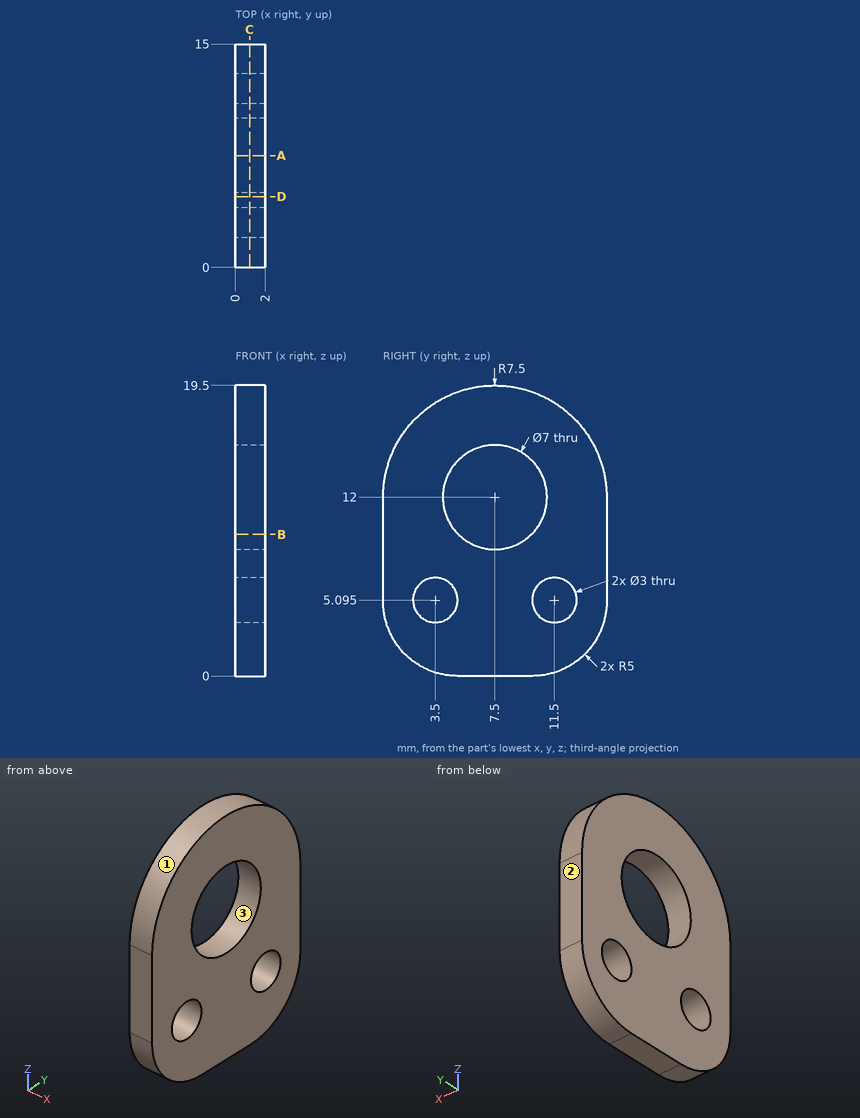
Study the drawing (mm; zero at the part's minimum x, y, z) and answer. Give positions to 0.01 mm unless a question says otherwise; leave off trailing zeros. Order: outer loops, then holes, each group sorted by start corner. A loop starts at its lowest first (then second) coordinate and runs counter-clockwise, first axis right, second up. Notation, with made-up numbers: (-2.5, 54.5) -> (37.5, 54.5) arc R29 cw to (37.5, 80.5) -> close; hole circle Ø8 at (43.5, 54.5). An arc over 180 degrees is marked (long way). Put each result on its own line as item: value.
Item 1: A cutting plane is placed at D-D on y = 4.75. Give the vertices of the cut face in (x, z) (1 decimal).
Established:
outline: (0, 0) -> (2, 0) -> (2, 4.3) -> (0, 4.3) -> close; (0, 5.9) -> (2, 5.9) -> (2, 9.8) -> (0, 9.8) -> close; (0, 14.2) -> (2, 14.2) -> (2, 19) -> (0, 19) -> close
Item 2: A cutting plane is placed at C-C on x = 0.95. Give the vertices of the cut face in (y, z) (3 decimals), plus the area to 3 significant figures.
Established:
outline: (0, 5) arc R5 ccw to (5, 0) -> (10, 0) arc R5 ccw to (15, 5) -> (15, 12) arc R7.5 ccw to (0, 12) -> close; hole circle Ø3 at (3.5, 5.095); hole circle Ø7 at (7.5, 12); hole circle Ø3 at (11.5, 5.095)
area: 205 mm^2
Item 3: A cutting plane is placed at A-A on y = 7.5. Give the vertices of the cut face in (x, z), plus the area to 3 significant figures.
Established:
outline: (0, 0) -> (2, 0) -> (2, 8.5) -> (0, 8.5) -> close; (0, 15.5) -> (2, 15.5) -> (2, 19.5) -> (0, 19.5) -> close
area: 25.0 mm^2
Item 4: For a pull along Y with two mould halves and no side action, classify the marked faces 1, 2 and 3 as released by +Y, released by -Y, zero draft, split by the parting line, or undercut.
Established:
face 1: split by the parting line
face 2: released by +Y
face 3: undercut
Item 5: Given P1, Ø3.5, axis at y = 11.5, z = 5.09, coming from the +X side; P2, Ø4, axis at y = 7.5, z = 12, coming from the -X side, each flat-ended and moving along its own axis, determine where each tip first touches the part or whether it passes through.
Established:
P1: stops at x = 2
P2: passes through
Item 6: A cutting plane is placed at B-B on z = 9.5. Give the vertices of the cut face in (x, y).
Established:
outline: (0, 0) -> (2, 0) -> (2, 5.05) -> (0, 5.05) -> close; (0, 9.95) -> (2, 9.95) -> (2, 15) -> (0, 15) -> close
Item 7: Straight lines are drawn through the part: line 1 (Y direction, x = 1.1, z = 12); line 2 (Z direction, x = 0.8, y = 10.25) (1 decimal); line 3 (Z direction, x = 0.8, y = 6). For each, find the intervals that lie inside material, in ascending order.
Established:
line 1: y = 0 to 4, 11 to 15
line 2: z = 0 to 4.3, 5.9 to 9.8, 14.2 to 19
line 3: z = 0 to 8.84, 15.16 to 19.35
